Here's how the part is built. I have some questions about the finished solid (model axes, mm). Give positions to 0.01 mm unless a question says otherwise; leave off trailing zeros. Loops run counter-clockwise (first coordinate to the right, second up) from the corner with the lowest first, then second, coordinate; pieces in that order, holes last. Notation, with made-up numbers: (76.25, 49) - (134.25, 49) arc R12 ccw to (134.25, 72) - close; hole circle Ø9 at (51.25, 45.5). An arc over 180 degrees is marked (long way). Use one line per item in the form item = value.
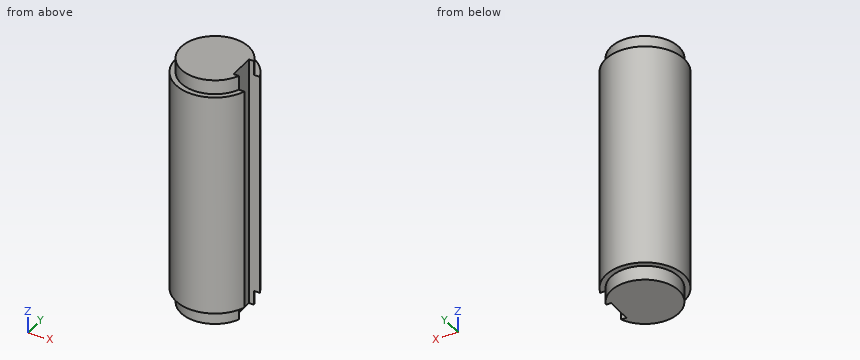
from build123d import *

# Parameters (mm, degrees)
SKETCH_R     = 15
PAD_DEPTH    = 86
SKETCH001_R  = 13
PAD001_DEPTH = 5.5
SKETCH002_R  = 13
PAD002_DEPTH = 5.5
SKETCH003_W  = 5
SKETCH003_H  = 10
POCKET_DEPTH = 117


with BuildPart() as part:
    # Sketch → Pad (new body)
    with BuildSketch(Plane.XY):
        Circle(SKETCH_R)
    extrude(amount=PAD_DEPTH)

    # Sketch001 (on Face3 of Pad) → Pad001 (join)
    with BuildSketch(Plane.XY.offset(86)):
        Circle(SKETCH001_R)
    extrude(amount=PAD001_DEPTH)

    # Sketch002 (on Face2 of Pad001) → Pad002 (join)
    with BuildSketch(Plane(origin=(0, 0, 0), x_dir=(1, 0, 0), z_dir=(0, 0, -1))):
        Circle(SKETCH002_R)
    extrude(amount=PAD002_DEPTH)

    # Sketch003 (on Face6 of Pad002) → Pocket (cut)
    with BuildSketch(Plane(origin=(0, 0, -5.5), x_dir=(1, 0, 0), z_dir=(0, 0, -1))):
        with Locations((12.5, 0)):
            Rectangle(SKETCH003_W, SKETCH003_H)
    extrude(amount=-POCKET_DEPTH, mode=Mode.SUBTRACT)


solid = part.part
(1) If I drill on probe 1 along Z at (x, y) = (9.5, -11.5); probe 2 along Y at (x, z) = (12.75, 46.5); probe 3 along X at (y, z) = (12, 87), over which ranges is the centre line in solid material (lowest first)?
Geometry says:
probe_1 = 0 to 86
probe_2 = -7.9 to -5, 5 to 7.9
probe_3 = -5 to 5
(2) For P1, Ø1.5, axis at x = 2.5, z = 30, coming from the -Y side; P2, Ø4.5, axis at x = 12, z = 57, coming from the +Y side; P3, Ø6, axis at x = 9, z = 21, coming from the -Y side, each with a flat end and sliding along its axis, tell me the tip position at first contact or that it passes through.
Geometry says:
P1 = -14.9
P2 = 11.4
P3 = -13.75
(3) If we section it at C-C (z = 71.5): List the corners of the cut face in (x, y) for me.
Geometry says:
outline = (10, -5) - (10, 5) - (14.14, 5) arc R15 ccw (long way) to (14.14, -5) - close
(4) If we section it at B-B (x = 0): List the corners of the cut face in (y, z) for me, plus the area to 3 significant figures.
Geometry says:
outline = (-15, 0) - (-13, 0) - (-13, -5.5) - (13, -5.5) - (13, 0) - (15, 0) - (15, 86) - (13, 86) - (13, 91.5) - (-13, 91.5) - (-13, 86) - (-15, 86) - close
area = 2,870 mm²
(5) If we section it at A-A (y = 0): List the corners of the cut face in (x, z) for me.
Geometry says:
outline = (-15, 0) - (-13, 0) - (-13, -5.5) - (10, -5.5) - (10, 91.5) - (-13, 91.5) - (-13, 86) - (-15, 86) - close
(6) If we section it at D-D (x = -8.5): List the corners of the cut face in (y, z) for me.
Geometry says:
outline = (-12.36, 0) - (-9.84, 0) - (-9.84, -5.5) - (9.84, -5.5) - (9.84, 0) - (12.36, 0) - (12.36, 86) - (9.84, 86) - (9.84, 91.5) - (-9.84, 91.5) - (-9.84, 86) - (-12.36, 86) - close
